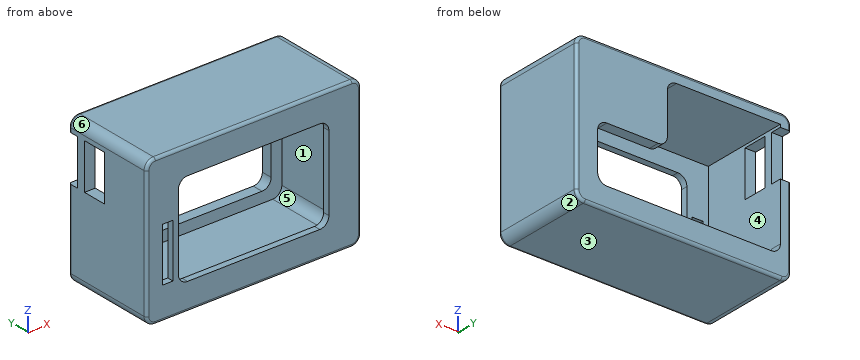
```python
from build123d import *

# Parameters (mm, degrees)
BOSS_EXTRUDE2_DEPTH = 14.4
SKETCH3_W           = 40.068
SKETCH3_H           = 27.368
SKETCH3_W_2         = 28.068
SKETCH3_H_2         = 17.368
BOSS_EXTRUDE3_DEPTH = 1.2
BOSS_EXTRUDE4_START = 14.4
SKETCH1_4_W         = 40.068
SKETCH1_4_H         = 27.368
BOSS_EXTRUDE4_DEPTH = 2
FILLET1_R           = 1.7
FILLET2_R           = 1.7
SKETCH4_W           = 8.5
SKETCH4_H           = 4.5
CUT_EXTRUDE1_DEPTH  = 2
SKETCH5_W           = 2
SKETCH5_H           = 10
CUT_EXTRUDE2_DEPTH  = 1.2
CUT_EXTRUDE3_DEPTH  = 2
FILLET4_R           = 1.7
SKETCH7_W           = 8.5
SKETCH7_H           = 2
CUT_EXTRUDE4_DEPTH  = 2
FILLET5_R           = 0.5


with BuildPart() as part:
    # Sketch1 → Boss-Extrude2 (new body)
    with BuildSketch(Plane(origin=(0, 0, 0), x_dir=(1, 0, 0), z_dir=(0, 1, 0))):
        Polygon((-20.034, 0), (-18.034, 0), (-18.034, 11.684), (0, 11.684), (0, 13.684), (-20.034, 13.684), align=None)
        Polygon((18.034, 11.684), (18.034, 0), (20.034, 0), (20.034, 13.684), (0, 13.684), (0, 11.684), align=None)
        Polygon((18.034, 0), (18.034, -11.684), (0, -11.684), (0, -13.684), (20.034, -13.684), (20.034, 0), align=None)
        Polygon((0, -13.684), (0, -11.684), (-18.034, -11.684), (-18.034, 0), (-20.034, 0), (-20.034, -13.684), align=None)
    extrude(amount=BOSS_EXTRUDE2_DEPTH)

    # Sketch3 → Boss-Extrude3 (add)
    with BuildSketch(Plane.XZ):
        Rectangle(SKETCH3_W, SKETCH3_H)
        Rectangle(SKETCH3_W_2, SKETCH3_H_2, mode=Mode.SUBTRACT)
    extrude(amount=BOSS_EXTRUDE3_DEPTH)

    # Sketch1<4> → Boss-Extrude4 (add)
    with BuildSketch(Plane(origin=(0, 0, 0), x_dir=(1, 0, 0), z_dir=(0, 1, 0)).offset(BOSS_EXTRUDE4_START)):
        Rectangle(SKETCH1_4_W, SKETCH1_4_H)
    extrude(amount=BOSS_EXTRUDE4_DEPTH)

    # Fillet1
    fillet1_edges = [part.edges().sort_by_distance(p)[0] for p in [
        (18.034, 7.2, -11.684),
        (-18.034, 7.2, -11.684),
        (18.034, 7.2, 11.684),
        (-20.034, 7.6, 13.684),
        (-20.034, 7.6, -13.684),
        (20.034, 7.6, -13.684),
        (20.034, 7.6, 13.684),
    ]]
    fillet(fillet1_edges, radius=FILLET1_R)

    # Fillet2
    fillet2_edges = [part.edges().sort_by_distance(p)[0] for p in [
        (14.034, -0.6, -8.684),
        (-14.034, -0.6, -8.684),
        (-14.034, -0.6, 8.684),
        (14.034, -0.6, 8.684),
    ]]
    fillet(fillet2_edges, radius=FILLET2_R)

    # Sketch4 → Cut-Extrude1 (cut)
    with BuildSketch(Plane.ZY.offset(20.034)):
        with Locations((6.934, 10.6)):
            Rectangle(SKETCH4_W, SKETCH4_H)
    extrude(amount=-CUT_EXTRUDE1_DEPTH, mode=Mode.SUBTRACT)

    # Sketch5 → Cut-Extrude2 (cut)
    with BuildSketch(Plane(origin=(0, 0, 0), x_dir=(-1, 0, 0), z_dir=(0, -1, 0))):
        with Locations((16.034, 2.684)):
            Rectangle(SKETCH5_W, SKETCH5_H)
    extrude(amount=CUT_EXTRUDE2_DEPTH, mode=Mode.SUBTRACT)

    # Sketch6 → Cut-Extrude3 (cut)
    with BuildSketch(Plane(origin=(0, 16.4, 0), x_dir=(1, 0, 0), z_dir=(0, 1, 0))):
        Polygon((-18.034, -11.684), (3.034, -11.684), (3.034, -0.684), (16.034, -0.684), (16.034, 9.684), (-18.034, 9.684), align=None)
    extrude(amount=-CUT_EXTRUDE3_DEPTH, mode=Mode.SUBTRACT)

    # Fillet4
    fillet4_edges = [part.edges().sort_by_distance(p)[0] for p in [
        (-18.034, 15.4, -9.684),
        (16.034, 15.4, -9.684),
        (16.034, 15.4, 0.684),
        (3.034, 15.4, 0.684),
        (3.034, 15.4, 11.684),
    ]]
    fillet(fillet4_edges, radius=FILLET4_R)

    # Sketch7 → Cut-Extrude4 (cut)
    with BuildSketch(Plane.ZY.offset(20.034)):
        with Locations((6.934, 15.4)):
            Rectangle(SKETCH7_W, SKETCH7_H)
    extrude(amount=-CUT_EXTRUDE4_DEPTH, mode=Mode.SUBTRACT)

    # Fillet5
    fillet5_edges = [part.edges().sort_by_distance(p)[0] for p in [
        (-20.034, 16.4, 11.584),
        (0, -1.2, 13.684),
        (0, 16.4, 13.684),
        (20.034, -1.2, 0),
        (-20.034, -1.2, 0),
        (0, -1.2, -13.684),
        (-19.536081528, -1.2, -13.186081528),
        (19.536081528, -1.2, -13.186081528),
        (19.536081528, -1.2, 13.186081528),
        (-19.536081528, -1.2, 13.186081528),
        (-20.034, 16.4, -4.65),
        (20.034, 16.4, 0),
        (0, 16.4, -13.684),
        (-19.536081528, 16.4, -13.186081528),
        (19.536081528, 16.4, -13.186081528),
        (19.536081528, 16.4, 13.186081528),
        (-19.536081528, 16.4, 13.186081528),
    ]]
    fillet(fillet5_edges, radius=FILLET5_R)


solid = part.part
```
CAD build for the part. Positions are in the model's coordinates, mm. Face numbers are marked on the shaded views. A direction names the side the tool comes from. Round coordinates to 2 decimals unless told otherwise and drop trailing zeros. Order: outer loops, then holes, each group sorted by start corner. A loop starts at its lowest first (then second) coordinate and runs counter-clockwise, first axis right, second up.
Item 1: Saw through at A-A on z = -6. Write the cut outline in (x, y).
Item 2: Mould opens along X. For the marked faces 1, 2, 3 and 4 say: pulls with the +X half, pulls with the -X half, needs draft (parallel to the pull), parting line crosses it, or undercut.
Item 3: Saw through at D-D on z = 6.25. Write the cut outline in (x, y), then the cut area to 3 significant figures.
Item 4: Pin check, flat tips, straight feed: pin 1 (0.6 mm diameter, centred on x = -19, z = 5.5, fed in from +Y); pin 2 (1 mm diameter, centred on y = -1, z = 1.5, fed in from +X); pin 3 (1.6 mm diameter, centred on x = -19.5, y = 15.5, fed in from -Z); pin 4 (2 mm diameter, centred on x = -19.5, y = 15.5, fed in from +Z). Stop position of each tip, or through.
Item 5: Probe line 1 along X through (y, z) = (11.5, -5); line 2 along X through (y, z) = (15, -2.5); line 3 along Z through (x, y) = (-10.5, 8). List the from-to ranges inside material, lowest first.
Item 6: Tool access for the marked faces 5 and 6: list every direction of +Z, -Z, +X, -X, +Y, -Y with a clear straight run to the whole face (end or side of a thin tool).
Item 7: Saw through at C-C on y = 5. Write the cut outline in (x, z).
Item 8: Saw through at B-B on x = -11.5. Write the cut outline in (y, z).
Reported:
1. outline: (-20.03, -0.7) arc R0.5 ccw to (-19.53, -1.2) - (-17.03, -1.2) - (-17.03, 0) - (-18.03, 0) - (-18.03, 16.4) - (-19.53, 16.4) arc R0.5 ccw to (-20.03, 15.9) - close; (-15.03, -1.2) - (-14.03, -1.2) - (-14.03, 0) - (-15.03, 0) - close; (14.03, -1.2) - (19.53, -1.2) arc R0.5 ccw to (20.03, -0.7) - (20.03, 15.9) arc R0.5 ccw to (19.53, 16.4) - (16.03, 16.4) - (16.03, 14.4) - (18.03, 14.4) - (18.03, 0) - (14.03, 0) - close
2. face 1: undercut
2. face 2: pulls with the +X half
2. face 3: needs draft
2. face 4: undercut
3. outline: (-20.03, -0.7) arc R0.5 ccw to (-19.53, -1.2) - (-14.03, -1.2) - (-14.03, 0) - (-18.03, 0) - (-18.03, 8.35) - (-20.03, 8.35) - close; (-20.03, 12.85) - (-18.03, 12.85) - (-18.03, 14.4) - (-20.03, 14.4) - close; (3.03, 14.4) - (18.03, 14.4) - (18.03, 0) - (14.03, 0) - (14.03, -1.2) - (19.53, -1.2) arc R0.5 ccw to (20.03, -0.7) - (20.03, 15.9) arc R0.5 ccw to (19.53, 16.4) - (3.03, 16.4) - close
3. area: 96.8 mm2
4. pin 1: stops at y = 14.4
4. pin 2: stops at x = 20.03
4. pin 3: stops at z = -13.64
4. pin 4: stops at z = 13.68
5. line 1: x = -20.03 to -18.03, 18.03 to 20.03
5. line 2: x = -20.03 to -18.03, 16.03 to 20.03
5. line 3: z = -13.68 to -11.68, 11.68 to 13.68
6. face 5: none
6. face 6: +Z, -X, +Y, -Y
7. outline: (-20.03, -11.98) arc R1.7 ccw to (-18.33, -13.68) - (18.33, -13.68) arc R1.7 ccw to (20.03, -11.98) - (20.03, 11.98) arc R1.7 ccw to (18.33, 13.68) - (-18.33, 13.68) arc R1.7 ccw to (-20.03, 11.98) - close; hole (-18.03, -9.98) arc R1.7 ccw to (-16.33, -11.68) - (16.33, -11.68) arc R1.7 ccw to (18.03, -9.98) - (18.03, 9.98) arc R1.7 ccw to (16.33, 11.68) - (-18.03, 11.68) - close
8. outline: (-1.2, -13.18) arc R0.5 ccw to (-0.7, -13.68) - (15.9, -13.68) arc R0.5 ccw to (16.4, -13.18) - (16.4, -9.68) - (14.4, -9.68) - (14.4, -11.68) - (0, -11.68) - (0, -8.68) - (-1.2, -8.68) - close; (-1.2, 8.68) - (0, 8.68) - (0, 11.68) - (16.4, 11.68) - (16.4, 13.18) arc R0.5 ccw to (15.9, 13.68) - (-0.7, 13.68) arc R0.5 ccw to (-1.2, 13.18) - close
